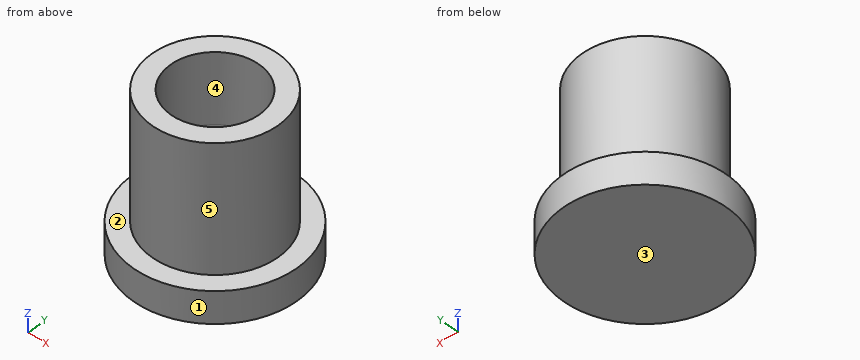
from build123d import *

# Parameters (mm, degrees)
F0_R     = 10
F0_R_2   = 13
F1_DEPTH = 5
F2_DEPTH = 25


with BuildPart() as f1:
    # F0 (on Top) → F1 (new body)
    with BuildSketch(Plane.XY):
        Circle(F0_R)
        Circle(F0_R_2)
        Circle(F0_R, mode=Mode.SUBTRACT)
    extrude(amount=F1_DEPTH)

    # F0 (on Top) → F2 (join)
    with BuildSketch(Plane.XY):
        Circle(F0_R)
    extrude(amount=F2_DEPTH)

    # F3 (on Front) → F4 (revolve, cut)
    with BuildSketch(Plane.XZ):
        with BuildLine():
            Line((7, 25), (0, 25))
            Line((0, 25), (0, 7))
            ThreePointArc((0, 7), (4.949747, 9.050253), (7, 14))
            Line((7, 14), (7, 25))
        make_face()
    revolve(axis=Axis((0, 0, 16), (0, 0, -1)), mode=Mode.SUBTRACT)


solid = f1.part
Geometry check sheet. Reference: the model listing, model coordinates, mm. Face numbers are marked on the shaded views. A direction names the side the tool comes from. Give positions to 0.01 mm unless a question says otherwise; leave off trailing zeros. Order: outer loops, then holes, each group sorted by start corner. A loop starts at its lowest first (then second) coordinate and runs counter-clockwise, first axis right, second up. Notation, with made-up numbers: (62, 86.25) - (83, 86.25) arc R33 cw to (83, 115.25) - close; hole circle Ø3 at (38.25, 68.25). An arc over 180 degrees is marked (long way). Answer as a JSON object with one key per item and string values.
(1) Draft check along X on the marked faces 3, 4 and 5. Enter one of: released by +X, released by -X, zero draft, split by the parting line, or undercut.
Report:
{"face 3": "zero draft", "face 4": "undercut", "face 5": "split by the parting line"}
(2) Cross-section at C-C (y = 9.5). Record the cut outline in (x, z).
Report:
{"outline": "(-8.87, 0) - (8.87, 0) - (8.87, 5) - (3.12, 5) - (3.12, 25) - (-3.12, 25) - (-3.12, 5) - (-8.87, 5) - close"}
(3) Cross-section at B-B (x = 8.5). Record the cut outline in (y, z), then the cut area to 3 significant figures.
Report:
{"outline": "(-9.84, 0) - (9.84, 0) - (9.84, 5) - (5.27, 5) - (5.27, 25) - (-5.27, 25) - (-5.27, 5) - (-9.84, 5) - close", "area": "309 mm^2"}
(4) Material ranges on line 1 (Y direction, x = 0, z = 18.75); line 2 (X direction, y = -0.25, z = 2.5); line 3 (X direction, y = 6, z = 18.25), recorded low to high.
Report:
{"line 1": "-10 to -7, 7 to 10", "line 2": "-13 to 13", "line 3": "-8 to -3.61, 3.61 to 8"}
(5) Cross-section at A-A (z = 23.25). Record the cut outline in (x, y).
Report:
{"outline": "circle Ø20 at (0, 0); hole circle Ø14 at (0, 0)"}
(6) Depth check by flat-ended pin: pin 1 Ø6 at (y, z) = (-6, 18) entering from +X; pin 2 Ø1 at (x, z) = (6.5, 10.5) entering from -Y; pin 3 Ø8 at (x, z) = (-9.5, 16) entering from +Y. Enter the tip coordinate at first touch or a pass-through.
Report:
{"pin 1": "x = 9.54", "pin 2": "y = -8", "pin 3": "y = 8.35"}
(7) Tool access check on the marked faces 1 and 2. Record the directions out of +Z, -Z, +X, -X, +Y, -Y that give a thin tool (end or side, any length) a straight path to the whole face; none if there is none.
Report:
{"face 1": "+Z, -Z", "face 2": "+Z"}
(8) Cross-section at D-D (z = 2.5). Record the cut outline in (x, y), then the cut area to 3 significant figures.
Report:
{"outline": "circle Ø26 at (0, 0)", "area": "531 mm^2"}
